```python
from build123d import *

# Parameters (mm, degrees)
F1_DEPTH = 3
F2_R     = 2
F3_R     = 2
F4_D     = 3.3
F5_R     = 15


with BuildPart() as f1:
    # F0 (on Top) → F1 (new body)
    with BuildSketch(Plane.XY):
        Polygon((110.177106271, 34.1935047355), (-49.822893729, 34.1935047355), (-49.822893729, -100.8064952645), (55.2746254304, -100.8064952645), (55.2746254304, -77.4659737945), (82.7258658507, -77.6009281682), (82.7258658507, -52.6009281682), (87.7258054305, -52.6255086135), (87.7258054305, -77.6009281682), (110.177106271, -77.7358825419), align=None)
    extrude(amount=F1_DEPTH)

    # F2
    f2_edges = [f1.edges().sort_by_distance(p)[0] for p in [
        (82.725866, -52.600928, 1.5),
    ]]
    fillet(f2_edges, radius=F2_R)

    # F3
    f3_edges = [f1.edges().sort_by_distance(p)[0] for p in [
        (87.725805, -52.625509, 1.5),
    ]]
    fillet(f3_edges, radius=F3_R)

    # F4 (through all)
    with Locations(Plane(origin=(0, 0, 0), x_dir=(1, 0, 0), z_dir=(0, 0, -1))):
        with Locations((-30.323264641, 90.3856833279), (35.2748671111, 90.7081734832)):
            Hole(F4_D / 2)

    # F5
    f5_edges = [f1.edges().sort_by_distance(p)[0] for p in [
        (110.177106, -77.735883, 1.5),
    ]]
    fillet(f5_edges, radius=F5_R)


solid = f1.part
```
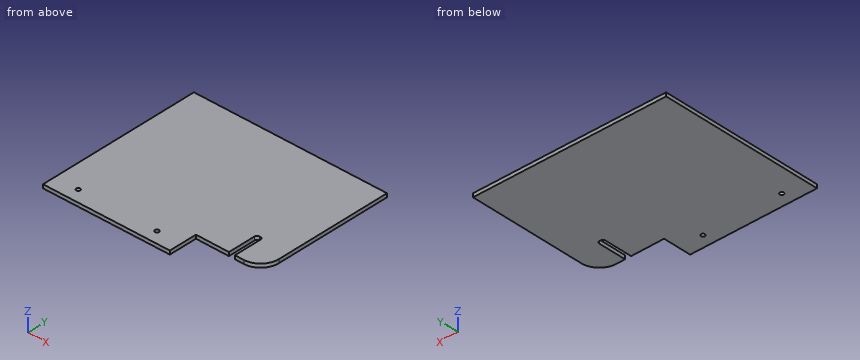
CAD build for the part. Positions are in the model's coordinates, mm. Round coordinates to 2 decimals unless told otherwise and drop trailing zeros. Order: outer loops, then holes, each group sorted by start corner. A loop starts at its lowest first (then second) coordinate and runs counter-clockwise, first axis right, second up.
Item 1: Saw through at B-B on y = -80. Write the cut outline in (x, z), then the cut area to 3 significant figures.
Item 2: Saw through at A-A on z = 1.65. Write the cut outline in (x, y), then the cut area to 3 significant figures.
Item 3: Pin check, flat tips, straight feed: pin 1 (2.5 mm diameter, centred on x = -30.32, y = -90.39, fed in from +Z); pin 2 (0.9 mm diameter, centred on y = -70.5, z = 1, fed in from +X); pin 3 (4 mm diameter, centred on x = 61, y = -55.5, fed in from -Z). Stop position of each tip, or through.
Item 4: Probe line 1 along X through (y, z) = (-57, 0.85); line 2 along Y through (x, z) = (-31, 1.95); line 3 along X through (y, z) = (-78.5, 2.7). List the from-to ranges inside material, lowest first.
Reported:
1. outline: (-49.82, 0) - (55.27, 0) - (55.27, 3) - (-49.82, 3) - close
1. area: 315 mm2
2. outline: (-49.82, -100.81) - (55.27, -100.81) - (55.27, -77.47) - (82.73, -77.6) - (82.73, -54.61) arc R2 cw to (84.74, -52.61) - (85.74, -52.62) arc R2 cw to (87.73, -54.62) - (87.73, -77.6) - (95.09, -77.65) arc R15 ccw to (110.18, -62.65) - (110.18, 34.19) - (-49.82, 34.19) - close; hole circle Ø3.3 at (-30.32, -90.39); hole circle Ø3.3 at (35.27, -90.71)
2. area: 20,100 mm2
3. pin 1: passes through
3. pin 2: stops at x = 108.22
3. pin 3: stops at z = 0
4. line 1: x = -49.82 to 82.73, 87.73 to 110.18
4. line 2: y = -100.81 to -91.89, -88.88 to 34.19
4. line 3: x = -49.82 to 55.27
